The drawing under review shows one solid part. Ordinate dimensions are in mm from its lowest x, y, z. Give positions to 0.01 mm unless a question says otherwise; leave off trailing zeros. Write each loop counter-clockwise with the first axis right and the second up, starting at its lowest first coordinate (ties: lowest second). Pieces come first, ordered by that corner, then holes. Notation, with made-up numbers: M 23.25,89 L 50.25,89 A13 ccw 50.25,99 Z; hole C -18.5,20.5 d10. An arc over 180 degrees is marked long. Write item = value, one per line. Start each with the question number.
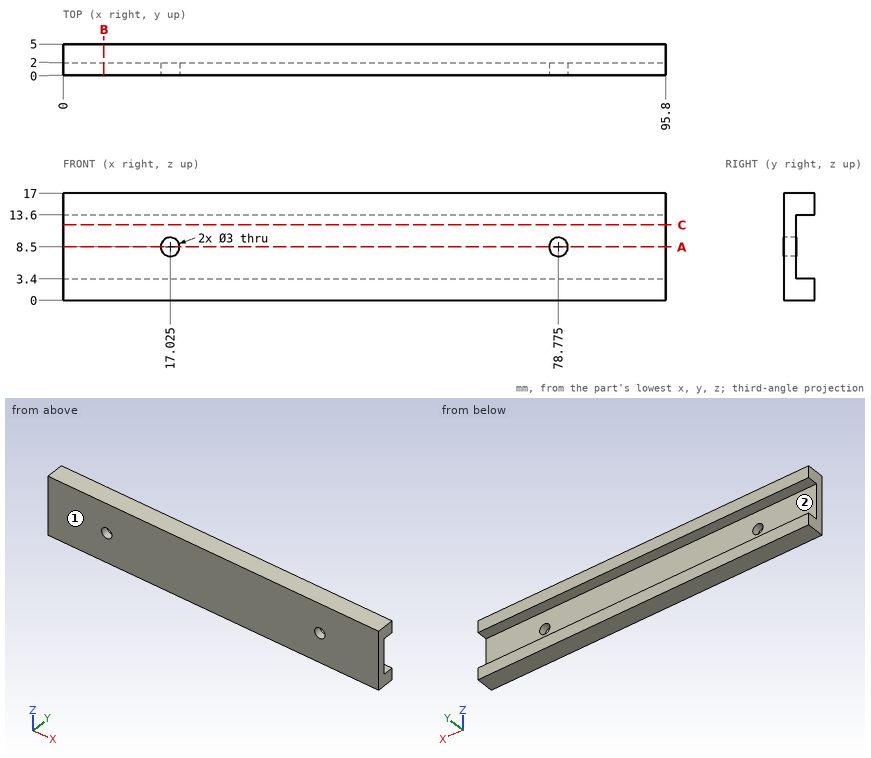
Item 1: Clearance check with flat-ended pins moving along their axes: P1, Ø3, axis at x = 33.5, z = 10.5, coming from the +Y side; P2, Ø1.8, axis at x = 78.775, z = 8.5, coming from the +Y side. State where each tip first meets the part, or that it passes through.
Item 2: We need section B-B, the plane x = 6.5. Write out the cut boundary in (y, z).
Item 3: To check wall thickness, follow probe 1 along X at (y, z) = (0.45, 8.5) (3 decimals); probe 2 along Z at (x, y) = (5.5, 3.5); probe 3 along Y at (x, z) = (12, 5.5). State the ranges of each line that lie inside material, in increasing order. Write a range as [from, to].
Item 4: The part is to be moulded in two halves that separate along Z. For the marked faces 1 and 2, say which applies: released by +Z, released by -Z, zero draft, split by the parting line, or undercut.
Item 5: We need section C-C, the plane z = 12. Write out the cut boundary in (x, y).
Item 6: We need section A-A, the plane z = 8.5. Write out the cut boundary in (x, y) (3 decimals), and give its area (3 significant figures).
Worked out:
q1.P1 = 2
q1.P2 = through
q2.outline = M 0,0 L 5,0 L 5,3.4 L 2,3.4 L 2,13.6 L 5,13.6 L 5,17 L 0,17 Z
q3.probe_1 = [0, 15.525], [18.525, 77.275], [80.275, 95.8]
q3.probe_2 = [0, 3.4], [13.6, 17]
q3.probe_3 = [0, 2]
q4.face_1 = zero draft
q4.face_2 = undercut
q5.outline = M 0,0 L 95.8,0 L 95.8,2 L 0,2 Z
q6.outline = M 0,0 L 15.525,0 L 15.525,2 L 0,2 Z; M 18.525,0 L 77.275,0 L 77.275,2 L 18.525,2 Z; M 80.275,0 L 95.8,0 L 95.8,2 L 80.275,2 Z
q6.area = 180 mm²
